Work out the finished part from the listing and answer in its coordinate system (mm). A direction names the side the tool comes from. Coordinates: 2 decimals unless noted, no trailing zeros. Loops run counter-clockwise (first coordinate to the right, second up) from the corner with the lowest first, then second, coordinate; pieces in that order, holes last. Notation, with made-up numbers: (-40, 12) -> (-1, 12) arc R16 cw to (-1, 18) -> close; hole circle Ø11 at (41, 0). An arc over 180 degrees is marked (long way). One line per question, with ' | ' between items.
```python
from build123d import *

# Parameters (mm, degrees)
F0_W     = 32
F0_H     = 32
F1_DEPTH = 2
F2_DEPTH = 15
F3_DEPTH = 2
F0_W_2   = 74
F0_H_2   = 2.5
F4_DEPTH = 10


with BuildPart() as f1:
    # F0 (on Top) → F1 (new body)
    with BuildSketch(Plane.XY):
        Polygon((6.5, -37), (37, -37), (37, -6.5), (37, 6.5), (37, 37), (-37, 37), (-37, -37), (-6.5, -37), align=None)
        with Locations((-18.5, -18.5)):
            Rectangle(F0_W, F0_H, mode=Mode.SUBTRACT)
        with Locations((18.5, -18.5)):
            Rectangle(F0_W, F0_H, mode=Mode.SUBTRACT)
        with Locations((-18.5, 18.5)):
            Rectangle(F0_W, F0_H, mode=Mode.SUBTRACT)
        with Locations((18.5, 18.5)):
            Rectangle(F0_W, F0_H, mode=Mode.SUBTRACT)
    extrude(amount=F1_DEPTH)



with BuildPart() as f2:
    # F0 (on Top) → F2 (new body)
    with BuildSketch(Plane.XY):
        Polygon((40, 79), (40, 6.5), (41, 6.5), (41, 80), (-41, 80), (-41, -80), (-6.5, -80), (-6.5, -79), (-40, -79), (-40, 79), align=None)
    extrude(amount=F2_DEPTH)


with BuildPart() as f2b:
    # F0 (on Top) → F2, piece 2 (new body)
    with BuildSketch(Plane.XY):
        Polygon((41, -6.5), (40, -6.5), (40, -79), (6.5, -79), (6.5, -80), (41, -80), align=None)
    extrude(amount=F2_DEPTH)


with BuildPart() as f1_1:
    add(f1.part)

    add(f2.part)  # F3 merges F2

    add(f2b.part)  # F3 merges F2b
    # F0 (on Top) → F3 (join)
    with BuildSketch(Plane.XY):
        Polygon((37, 37), (37, 6.5), (40, 6.5), (40, 79), (-40, 79), (-40, -79), (-6.5, -79), (-6.5, -76.5), (-9, -76.5), (-37, -76.5), (-37, -39.5), (-37, -37), (-37, 37), (-37, 39.5), (-37, 76.5), (37, 76.5), (37, 39.5), align=None)
        Polygon((37, -6.5), (37, -37), (37, -39.5), (37, -76.5), (9, -76.5), (6.5, -76.5), (6.5, -79), (40, -79), (40, -6.5), align=None)
    extrude(amount=F3_DEPTH)

    # F0 (on Top) → F4 (join)
    with BuildSketch(Plane.XY):
        Polygon((-6.5, -76.5), (-6.5, -37), (-37, -37), (-37, -39.5), (-9, -39.5), (-9, -76.5), align=None)
        Polygon((37, -39.5), (37, -37), (6.5, -37), (6.5, -76.5), (9, -76.5), (9, -39.5), align=None)
        with Locations((0, 38.25)):
            Rectangle(F0_W_2, F0_H_2)
    extrude(amount=F4_DEPTH)


solid = f1_1.part
```
1) Flat-ended cylindrical pins translate along their axes: pin 1 (1.2 mm diameter, centred on x = 17, y = 38.5, fed in from +Z); pin 2 (2 mm diameter, centred on x = 0, z = 1, fed in from -Y). Find the tip coordinate at first contact, or state that the pin passes through.
Check values:
pin 1: stops at z = 10 | pin 2: stops at y = -37
2) For faces 4 (the face through (40, 43, 8)), 5 (the face through (23, -39.5, 5)), 6 (the face through (41, -44, 7)), determine the directions among +Z, -Z, +X, -X, +Y, -Y from which every point of the face is accessible in a straight line to the end or side of a thin tool.
Check values:
face 4: +Z | face 5: +Z, -Z | face 6: +Z, -Z, +X, +Y, -Y
3) Find the intervals of material crossed by line 1 along Y through (x, z) = (36.5, 3.75); line 2 along X through (y, z) = (-42.5, 0.5); line 3 along Y through (x, z) = (29, 0.5), in increasing order.
Check values:
line 1: y = -80 to -79, -39.5 to -37, 37 to 39.5, 79 to 80 | line 2: x = -41 to -37, -9 to -6.5, 6.5 to 9, 37 to 41 | line 3: y = -80 to -76.5, -39.5 to -34.5, -2.5 to 2.5, 34.5 to 39.5, 76.5 to 80
4) Find section A-A (y = 59). Write down the section's boundary in (x, z), plus the area to 3 significant figures.
Check values:
outline: (-41, 0) -> (-37, 0) -> (-37, 2) -> (-40, 2) -> (-40, 15) -> (-41, 15) -> close; (37, 0) -> (41, 0) -> (41, 15) -> (40, 15) -> (40, 2) -> (37, 2) -> close | area: 42.0 mm^2
5) Find section D-D (y = -63.5). Write down the section's boundary in (x, z).
Check values:
outline: (-41, 0) -> (-37, 0) -> (-37, 2) -> (-40, 2) -> (-40, 15) -> (-41, 15) -> close; (-9, 0) -> (-6.5, 0) -> (-6.5, 10) -> (-9, 10) -> close; (6.5, 0) -> (9, 0) -> (9, 10) -> (6.5, 10) -> close; (37, 0) -> (41, 0) -> (41, 15) -> (40, 15) -> (40, 2) -> (37, 2) -> close
6) Find section C-C (z = 3.75). State how many separate pieces and enclosed holes the cut face has, plus the area to 4 significant figures.
Check values:
separate pieces: 5 | enclosed holes: 0 | area: 976.5 mm^2
7) Find section B-B (x = 0.5). Write down the section's boundary in (y, z), plus the area to 3 significant figures.
Check values:
outline: (-37, 0) -> (39.5, 0) -> (39.5, 10) -> (37, 10) -> (37, 2) -> (-37, 2) -> close; (76.5, 0) -> (80, 0) -> (80, 15) -> (79, 15) -> (79, 2) -> (76.5, 2) -> close | area: 193 mm^2
8) The mould has two halves that part along Y. Classify faces 1 (the face through (-1, 37, 6)), 2 (the face through (-24, -80, 7)), 3 (the face through (-41, 1, 7)): released by +Y, released by -Y, zero draft, split by the parting line, or undercut.
Check values:
face 1: undercut | face 2: released by -Y | face 3: zero draft
